Here's the drawing with two shaded views (mm, measured from the low corner). I have some questions. Coordinates: 2 decimals unless noted, no trailing zeros. Write each loop counter-clockwise with the first axis right and the second up, starting at its lowest first coordinate (ties: lowest second). Pieces come first, ordered by that corner, then holes. Notation, with made-up numbers: (49.5, 41) -> (90.5, 41) arc R29 cw to (90.5, 63) -> close; hole circle Ø6 at (9.25, -3.75). An arc over 180 degrees is marked (long way). Use a Markdown table: item, result. Add a question column.
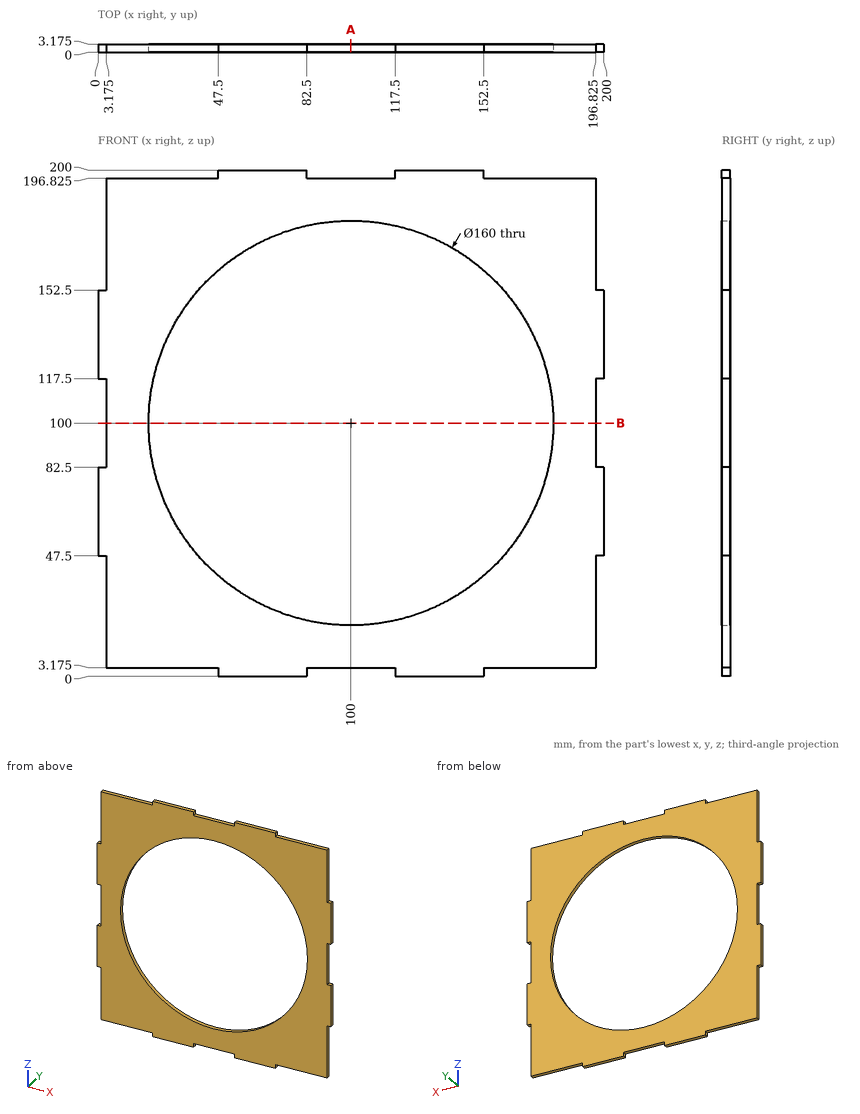
Q1. Please list where these lines run through material, in increasing order: line 1 (X direction, y = 1.15, z = 100) (3 decimals); line 2 (X direction, y = 1.4, z = 189) (3 decimals).
Q2. Suppose I cut it at B-B, the plane z = 100. Write out the boundary of the cut face in (x, y) (3 decimals).
Q3. Suppose I cut it at A-A, the plane x = 100. Write out the boundary of the cut face in (y, z) (3 decimals), and give its area (3 significant figures).
Q4. Will these pins go through, and if not, where does the flat tip stop? pin 1 (1.6 mm diameter, centred on x = 1, y = 1.5, fed in from +Z); pin 2 (1.6 mm diameter, centred on x = 199, y = 2, fed in from -Z); pin 3 (1 mm diameter, centred on y = 1.5, z = 27, fed in from -X) (3 decimals).
Answer key:
| question | item | result |
|---|---|---|
| 1 | line 1 | x = 3.175 to 20, 180 to 196.825 |
| 1 | line 2 | x = 3.175 to 196.825 |
| 2 | outline | (3.175, 0) -> (20, 0) -> (20, 3.175) -> (3.175, 3.175) -> close; (180, 0) -> (196.825, 0) -> (196.825, 3.175) -> (180, 3.175) -> close |
| 3 | outline | (0, 3.175) -> (3.175, 3.175) -> (3.175, 20) -> (0, 20) -> close; (0, 180) -> (3.175, 180) -> (3.175, 196.825) -> (0, 196.825) -> close |
| 3 | area | 107 mm^2 |
| 4 | pin 1 | stops at z = 152.5 |
| 4 | pin 2 | stops at z = 47.5 |
| 4 | pin 3 | stops at x = 3.175 |
